Can you work these out from the drawing? Everything is in mm from the part's minimum corner. A direction names the side the tool comes from. Round coordinates to 2 decimals unless told otherwise and drop trailing zeros. Loops run counter-clockwise (first coordinate to the right, second up) from the corner with the lowest first, then second, coordinate; pieces in that order, holes last. Notation, with made-up numbers: (29.25, -32.5) -> (41.25, -32.5) arc R13 ccw to (41.25, -8.5) -> close; hole circle Ø8 at (49.5, 22). An arc over 180 degrees is marked (long way). One line per item, written item: value.
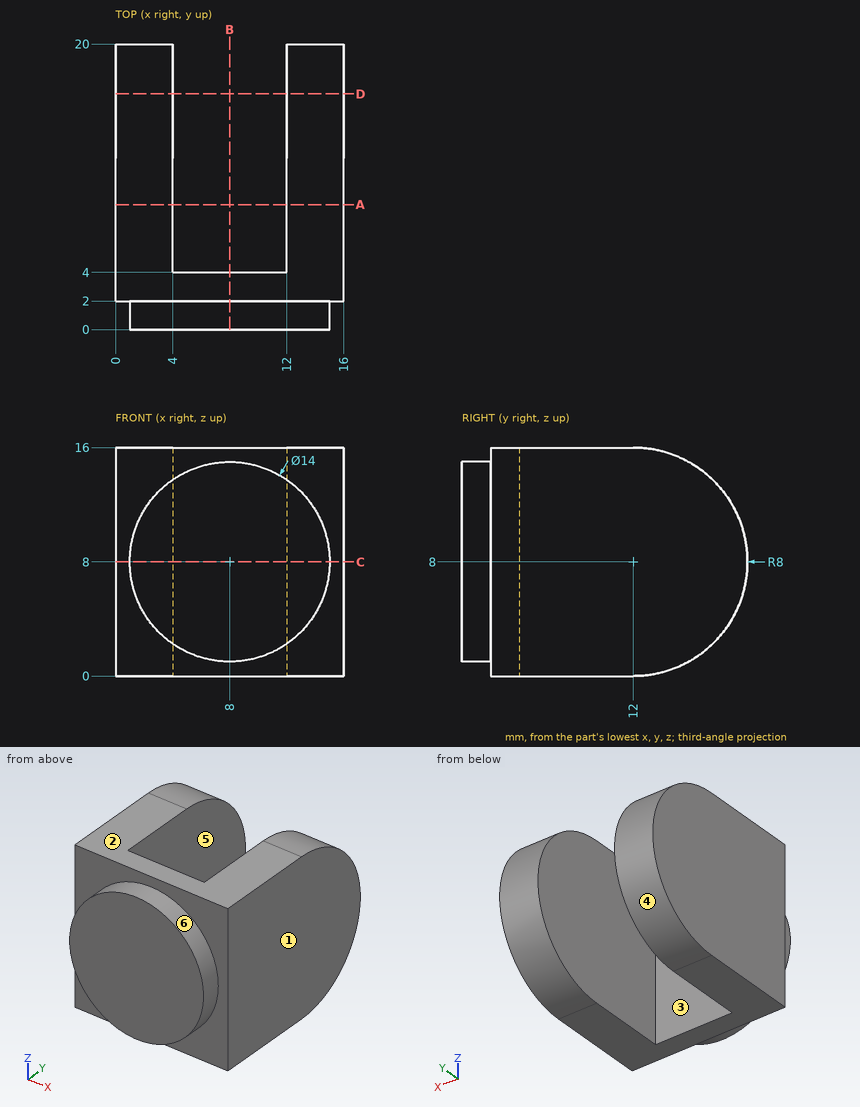
Item 1: If we mould it in two halves opening along X, with no side actions, what happens to the marked faces 1, 2 and 3? For each: released by +X, released by -X, zero draft, split by the parting line, or undercut.
Output:
face 1: released by +X
face 2: zero draft
face 3: undercut
Item 2: For the marked faces 4, 5 and 6, which set-ups out of +Z, -Z, +X, -X, +Y, -Y let a thin tool reach every point of the face, with its end or its side?
Output:
face 4: +X, -X, +Y
face 5: +Z, -Z, +Y
face 6: -Y
Item 3: Will these pins go through, and if not, where does the flat tip stop? pin 1 Ø1.5 at (y, z) = (7, 4) entering from -X; pin 2 Ø2 at (x, z) = (9, 7.5) entering from +Y.
Output:
pin 1: stops at x = 0
pin 2: stops at y = 4
Item 4: If we section it at C-C on z = 8: List the corners of the cut face in (x, y) for me.
Output:
outline: (0, 2) -> (1, 2) -> (1, 0) -> (15, 0) -> (15, 2) -> (16, 2) -> (16, 20) -> (12, 20) -> (12, 4) -> (4, 4) -> (4, 20) -> (0, 20) -> close
Item 5: I need wall thicknesses on line 1 (X direction, y = 17, z = 7.5); line 2 (Y direction, x = 5.5, z = 1.75); line 3 (Y direction, x = 2.75, z = 2). Which ranges of each line are inside material? Lowest first, please. Write a range as from..to.
Output:
line 1: x = 0..4, 12..16
line 2: y = 0..4
line 3: y = 2..17.29
Item 6: If we section it at D-D on y = 16.5: List the corners of the cut face in (x, z) for me, plus the area to 3 significant figures.
Output:
outline: (0, 1.39) -> (4, 1.39) -> (4, 14.61) -> (0, 14.61) -> close; (12, 1.39) -> (16, 1.39) -> (16, 14.61) -> (12, 14.61) -> close
area: 106 mm²
Item 7: If we section it at A-A on y = 8.75: List the corners of the cut face in (x, z) for me.
Output:
outline: (0, 0) -> (4, 0) -> (4, 16) -> (0, 16) -> close; (12, 0) -> (16, 0) -> (16, 16) -> (12, 16) -> close
Item 8: If we section it at B-B on x = 8: List the corners of the cut face in (y, z) for me.
Output:
outline: (0, 1) -> (2, 1) -> (2, 0) -> (4, 0) -> (4, 16) -> (2, 16) -> (2, 15) -> (0, 15) -> close
